```python
from build123d import *

# Parameters (mm, degrees)
SKETCH_W                = 60
SKETCH_H                = 30
PAD_DEPTH               = 3.5
POCKET_DEPTH            = 30.001
LINEARPATTERN_COUNT     = 4
LINEARPATTERN_PITCH     = 15
SKETCH002_W             = 10
SKETCH002_H             = 12.5
SKETCH002_W_2           = 60
SKETCH002_H_2           = 3.5
PAD001_DEPTH            = 2
SKETCH003_R             = 1.3
PAD002_DEPTH            = 2
SKETCH004_W             = 10
SKETCH004_H             = 2
PAD003_DEPTH            = 3
SKETCH005_W             = 10
SKETCH005_H             = 1.6
PAD004_DEPTH            = 1
SKETCH005_MIRRORED_2_W  = 10
SKETCH005_MIRRORED_2_H  = 1.6
PAD004_MIRRORED_2_DEPTH = 1
CHAMFER_SIZE            = 0.8
CHAMFER001_SIZE         = 0.3


with BuildPart() as part:
    # Sketch → Pad (new body)
    with BuildSketch(Plane.XY):
        Rectangle(SKETCH_W, SKETCH_H)
    extrude(amount=PAD_DEPTH)

    # Sketch001 (on Face3 of Pad) → Pocket (cut, through all)
    with BuildSketch(Plane.XZ.offset(15)):
        with BuildLine():
            Line((-24, 0.722949), (-24, 0))
            Line((-24, 0), (-21, 0))
            Line((-21, 0), (-21, 0.722949))
            ThreePointArc((-21, 0.722949), (-20.37226, 1.668412), (-20.285841, 2.8))
            Line((-24.714159, 2.8), (-20.285841, 2.8))
            ThreePointArc((-24.714159, 2.8), (-24.62774, 1.668412), (-24, 0.722949))
        make_face()
    pocket = extrude(amount=-POCKET_DEPTH, mode=Mode.SUBTRACT)

    # LinearPattern: Pocket ×4
    with Locations(*[(i * LINEARPATTERN_PITCH, 0, 0) for i in range(1, LINEARPATTERN_COUNT)]):
        add(pocket, mode=Mode.SUBTRACT)

    # Sketch002 (on Face28 of LinearPattern) → Pad001 (join)
    with BuildSketch(Plane.XY.offset(3.5)):
        with Locations((-25, 8.75)):
            Rectangle(SKETCH002_W, SKETCH002_H)
        with Locations((0, -13.25)):
            Rectangle(SKETCH002_W_2, SKETCH002_H_2)
        with Locations((25, 8.75)):
            Rectangle(SKETCH002_W, SKETCH002_H)
    extrude(amount=PAD001_DEPTH)

    # Sketch003 (on Face37 of Pad001) → Pad002 (join)
    with BuildSketch(Plane.XY.offset(5.5)):
        with Locations((-25, 7.5)):
            Circle(SKETCH003_R)
        with Locations((25, 7.5)):
            Circle(SKETCH003_R)
    extrude(amount=PAD002_DEPTH)

    # Sketch004 (on Face37 of Pad002) → Pad003 (join)
    with BuildSketch(Plane.XY.offset(5.5)):
        with Locations((-25, 14)):
            Rectangle(SKETCH004_W, SKETCH004_H)
        with Locations((25, 14)):
            Rectangle(SKETCH004_W, SKETCH004_H)
        with Locations((-25, -14)):
            Rectangle(SKETCH004_W, SKETCH004_H)
        with Locations((25, -14)):
            Rectangle(SKETCH004_W, SKETCH004_H)
    extrude(amount=PAD003_DEPTH)

    # Sketch005 (on Face65 of Pad003) → Pad004 (join)
    with BuildSketch(Plane.XZ.offset(-13)):
        with Locations((-25, 7.7)):
            Rectangle(SKETCH005_W, SKETCH005_H)
    pad004 = extrude(amount=PAD004_DEPTH)

    # Sketch005 Mirrored 2 → Pad004 Mirrored 2 (add)
    with BuildSketch(Plane(origin=(0, 13, 0), x_dir=(-1, 0, 0), z_dir=(0, 1, 0))):
        with Locations((-25, 7.7)):
            Rectangle(SKETCH005_MIRRORED_2_W, SKETCH005_MIRRORED_2_H)
    pad004_mirrored_2 = extrude(amount=-PAD004_MIRRORED_2_DEPTH)

    # Mirrored001: Pad004, Pad004 Mirrored 2 across XZ
    add(pad004.mirror(Plane.XZ))
    add(pad004_mirrored_2.mirror(Plane.XZ))

    # Chamfer
    chamfer_edges = [part.edges().sort_by_distance(p)[0] for p in [
        (-25, -12, 6.9),
        (25, -12, 6.9),
        (-25, 12, 6.9),
        (25, 12, 6.9),
    ]]
    chamfer(chamfer_edges, length=CHAMFER_SIZE)

    # Chamfer001
    chamfer001_edges = [part.edges().sort_by_distance(p)[0] for p in [
        (25, 12, 8.5),
        (-25, 12, 8.5),
        (25, -12, 8.5),
        (-25, -12, 8.5),
    ]]
    chamfer(chamfer001_edges, length=CHAMFER001_SIZE)


solid = part.part
```
Model file for the job. Use its own axes, mm. A direction names the side the tool comes from. Coordinates: 2 decimals unless noted, no trailing zeros. Loops run counter-clockwise (first coordinate to the right, second up) from the corner with the lowest first, then second, coordinate; pieces in that order, holes last. Notation, with made-up numbers: M 30,80.5 L 87,80.5 A13 cw 87,103.5 Z; hole C 56,4.5 d4. An arc over 180 degrees is marked long. Use CSV: the item, a comma, the result in double quotes. Start each with the question number.
1. Band-saw the part on A-A, the plane z = 2. List the corners of the cut face in (x, y).
2. Flat gauge pins, fed straight in: pin 1 (8 mm diameter, centred on x = -7.5, y = -2.5, fed in from +Z); pin 2 (0.8 mm diameter, centred on x = 25.5, y = 7.5, fed in from +Z). Where does each tip first touch, or does it go through?
3. Band-saw the part on B-B, the plane z = 6.25. List the corners of the cut face in (x, y), then the cut area to 3 significant figures.
4. Band-saw the part on D-D, the plane x = -14. List the corners of the cut face in (y, z).
5. Probe probe 1 along X at (y, z) = (7, 2.5); probe 2 along X at (y, z) = (9.5, 4.75); probe 3 along X at (y, z) = (-9, 0.5). List the from-to ranges inside material, lowest first. Write a range as [from, to].
6. Two-plate mould, pull along Z, no slides. Class faces 1 (the flat face through (22, 0, 2.8)), 2 (the flat face through (-25, 14, 8.5)), 3 (the cylindrical face through (23.7, 7.56, 6.49)): pulls with the +Z half, pulls with the -Z half, needs draft (parallel to the pull), parting line crosses it, or undercut.
7. Tool access for faces 4 (the flat face through (0, -13, 5.5)), 5 (the flat face through (20, -14, 7)), 6 (the cylindrical face through (-5.38, -0.21, 1.65)), 7 (the flat face through (25, 2.5, 4)): list every direction of +Z, -Z, +X, -X, +Y, -Y with a clear straight run to the whole face (end or side of a thin tool).
Entries:
1,outline,"M -30,-15 L -24.71,-15 L -24.71,15 L -30,15 Z; M -20.29,-15 L -9.71,-15 L -9.71,15 L -20.29,15 Z; M -5.29,-15 L 5.29,-15 L 5.29,15 L -5.29,15 Z; M 9.71,-15 L 20.29,-15 L 20.29,15 L 9.71,15 Z; M 24.71,-15 L 30,-15 L 30,15 L 24.71,15 Z"
2,pin 1,"stops at z = 3.5"
2,pin 2,"stops at z = 7.5"
3,outline,"M -30,-15 L -20,-15 L -20,-13 L -30,-13 Z; M -30,13 L -20,13 L -20,15 L -30,15 Z; C -25,7.5 d2.6; M 20,-15 L 30,-15 L 30,-13 L 20,-13 Z; M 20,13 L 30,13 L 30,15 L 20,15 Z; C 25,7.5 d2.6"
3,area,"90.6 mm2"
4,outline,"M -15,0 L 15,0 L 15,3.5 L -11.5,3.5 L -11.5,5.5 L -15,5.5 Z"
5,probe 1,"x = [-30, -24.75], [-20.25, -9.75], [-5.25, 5.25], [9.75, 20.25], [24.75, 30]"
5,probe 2,"x = [-30, -20], [20, 30]"
5,probe 3,"x = [-30, -24], [-21, -9], [-6, 6], [9, 21], [24, 30]"
6,face 1,"undercut"
6,face 2,"pulls with the +Z half"
6,face 3,"needs draft"
7,face 4,"none"
7,face 5,"+Z, +Y, -Y"
7,face 6,"+Y, -Y"
7,face 7,"+Z, +X, -X"
